Answer from the drawing. Dimensions are ordinates in mm from the lowest x, y and z of the part. A direction names the side the tool comes from. Round coordinates to 2 decimals unless told otherwise and drop trailing zeros. Loops run counter-clockwise (first coordinate to the right, second up) from the corner with the lowest first, then second, coordinate; pieces in that order, holes last.
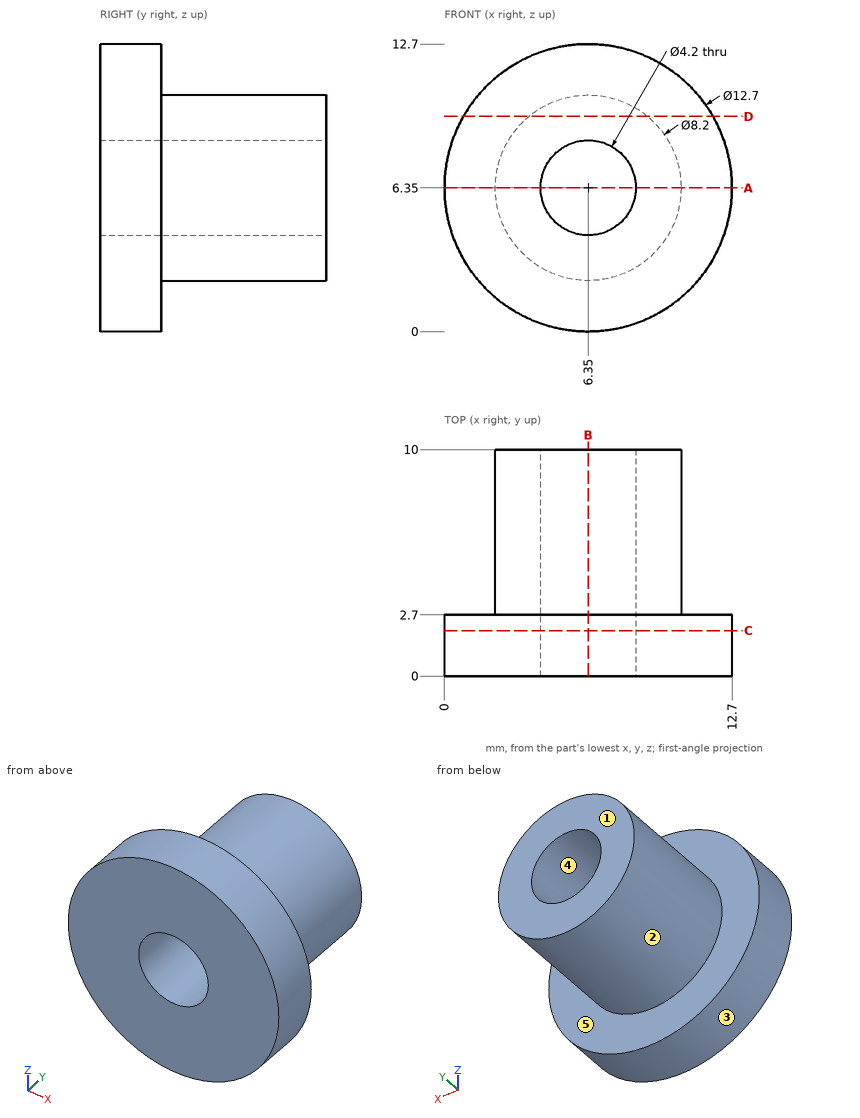
Item 1: Section C-C, the plane y = 2 is taken. Give the vertices of the cut face in (x, z).
Item 2: Section B-B, the plane x = 6.35 is taken. Give the vertices of the cut face in (y, z), plus the area to 4 significant figures.
Item 3: Straight lines are drawn through the part: line 1 (Z direction, x = 6.35, y = 3.25); line 2 (Y direction, x = 6, z = 1.5). For each, find the intervals that lie inside material, in ascending order.
Item 4: For the marked faces 1 and 2, determine the directions among +Z, -Z, +X, -X, +Y, -Y from which every point of the face is accessible in a straight line to the end or side of a thin tool.
Item 5: Section D-D, the plane z = 9.5 is taken. Give the vertices of the cut face in (x, y), plus the area to 3 significant figures.
Item 6: Determine the mould class of the marked faces 3, 4 and 5 for opening direction X: pulls with the +X half, pulls with the -X half, needs draft (parallel to the pull), parting line crosses it, or undercut.
Item 7: Section A-A, the plane z = 6.35 is taken. Give the vertices of the cut face in (x, y).
Item 8: Each of these flat-tipped pins is pushed along its axis until it touches: P1, Ø1.5, axis at x = 3, y = 7, coming from the -Z side; P2, Ø4, axis at x = 5, y = 6, coming from the +Z side; P3, Ø2, axis at x = 9, y = 2.5, coming from the +Z side; P4, Ø4, axis at x = 6, z = 8, coming from the +Y side. Where does it stop, or does it pass through?
Answer below:
1. outline: circle Ø12.7 at (6.35, 6.35); hole circle Ø4.2 at (6.35, 6.35)
2. outline: (0, 0) - (2.7, 0) - (2.7, 2.25) - (10, 2.25) - (10, 4.25) - (0, 4.25) - close; (0, 8.45) - (10, 8.45) - (10, 10.45) - (2.7, 10.45) - (2.7, 12.7) - (0, 12.7) - close
2. area: 52.15 mm2
3. line 1: z = 2.25 to 4.25, 8.45 to 10.45
3. line 2: y = 0 to 2.7
4. face 1: +Z, -Z, +X, -X, +Y
4. face 2: +Y
5. outline: (0.84, 0) - (11.86, 0) - (11.86, 2.7) - (8.97, 2.7) - (8.97, 10) - (3.73, 10) - (3.73, 2.7) - (0.84, 2.7) - close
5. area: 68.1 mm2
6. face 3: parting line crosses it
6. face 4: undercut
6. face 5: needs draft
7. outline: (0, 0) - (4.25, 0) - (4.25, 10) - (2.25, 10) - (2.25, 2.7) - (0, 2.7) - close; (8.45, 0) - (12.7, 0) - (12.7, 2.7) - (10.45, 2.7) - (10.45, 10) - (8.45, 10) - close
8. P1: stops at z = 3.18
8. P2: stops at z = 10.45
8. P3: stops at z = 12.48
8. P4: stops at y = 10
